```python
from build123d import *

# Parameters (mm, degrees)
F0_W   = 14.125
F0_H   = 3
F0_W_2 = 9.875
F0_H_2 = 2
F0_W_3 = 1
F2_R   = 1
F3_R   = 5
F4_R   = 2


with BuildPart() as f1:
    # F0 (on Front) → F1 (revolve)
    with BuildSketch(Plane.XZ):
        Polygon((-14.875, -9.095676), (-14.875, 34.029324), (-15.875, 34.029324), (-15.875, -20.970676), (-14.875, -20.970676), (-14.875, -18.970676), align=None)
        with Locations((-22.9375, 35.529324)):
            Rectangle(F0_W, F0_H)
        with Locations((-9.9375, -19.970676)):
            Rectangle(F0_W_2, F0_H_2)
        with Locations((-15.375, 35.529324)):
            Rectangle(F0_W_3, F0_H)
        with BuildLine():
            ThreePointArc((-5, -18.970676), (-11.982679, -16.078356), (-14.875, -9.095676))
            Line((-14.875, -9.095676), (-14.875, -18.970676))
            Line((-14.875, -18.970676), (-5, -18.970676))
        make_face()
    revolve(axis=Axis((0, 0, 3.538087), (0, 0, -1)))

    # F2
    f2_edges = [f1.edges().sort_by_distance(p)[0] for p in [
        (5, 0, -20.970676),
        (5, 0, -18.970676),
        (15.875, 0, -20.970676),
    ]]
    fillet(f2_edges, radius=F2_R)

    # F3
    f3_edges = [f1.edges().sort_by_distance(p)[0] for p in [
        (14.875, 0, 37.029324),
    ]]
    fillet(f3_edges, radius=F3_R)

    # F4
    f4_edges = [f1.edges().sort_by_distance(p)[0] for p in [
        (30, 0, 37.029324),
    ]]
    fillet(f4_edges, radius=F4_R)


solid = f1.part
```
CAD build for the part. Positions are in the model's coordinates, mm. A direction names the side the tool comes from. Give positions to 0.01 mm unless a question says otherwise; leave off trailing zeros. Write each loop counter-clockwise with the first axis right and the second up, starting at its lowest first coordinate (ties: lowest second). Pieces come first, ordered by that corner, then holes. Notation, with made-up numbers: M -14,46.5 L 39,46.5 A25 cw 39,58.5 Z; hole C -25.75,77 d9. An arc over 180 degrees is marked long. Return JSON: item names as keys, results as strings. Group by question number.
(1) Drill centre lines: L1, parallel to Y at x = 0, z = -19.95 (3 decimals); L2, parallel to Z at x = -24.5, y = 1; L3, parallel to Y at x = 0, z = 17 (3 decimals). Where is each one in solid material? Low to high. Write a range as [from, to].
(2) 3-axis set-ups, long thin cutter, end or side, ignore diameter. For faces 1 (the face through (3.441, -15.497, 6.651)), 2 (the face through (-6.4, 0.2, -20.971)): which of +Z, -Z, +X, -X, +Y, -Y reach the whole face in a straight line?
(3) Flat gauge pins, fed straight in: pin 1 Ø3 at (x, z) = (6.5, -13.5) entering from -Y; pin 2 Ø12 at (y, z) = (-18.5, 13.5) entering from +X; pin 3 Ø1.5 at (x, y) = (-8.5, 16) entering from -Z. Where does each tip first touch, or does it go through?
(4) Mould opens along X. For faces 3 (the face through (-13, -13, 34.029)), 4 (the face through (29.97, 1.32, 34.54)), 5 (the face through (-8, 12.54, 11.75)) say: pulls with the +X half, pulls with the -X half, needs draft (parallel to the pull), parting line crosses it, or undercut.
(5) Band-saw the part on A-A (z = 24.5). Give the cut face in (x, y) (3 decimals).
Entries:
{
 "1": {"L1": "y = [-15.875, -5], [5, 15.875]", "L2": "z = [34.03, 37.03]", "L3": "y = [-15.875, -14.875], [14.875, 15.875]"},
 "2": {"face 1": "-Z", "face 2": "-Z, +X, -X, +Y, -Y"},
 "3": {"pin 1": "stops at y = -15.07", "pin 2": "stops at x = 9.79", "pin 3": "stops at z = 34.03"},
 "4": {"face 3": "needs draft", "face 4": "parting line crosses it", "face 5": "undercut"},
 "5": {"outline": "C 0,0 d31.75; hole C 0,0 d29.75"}
}
